Build history of the part. All positions in model axes, mm. A direction names the side the tool comes from. Give positions to 0.01 mm unless a question says otherwise; leave off trailing zeros. Order: outer loops, then holes, each group sorted by start corner. A loop starts at its lowest first (then second) coordinate and runs counter-clockwise, first axis right, second up. Notation, with made-up numbers: M 51.5,-24 L 92.5,-24 A10 cw 92.5,-6 Z; hole C 83.25,56.25 d2. An arc over 180 degrees is marked long. Use CSV: the item, a comma, the result in double quotes. Start each with the question number.
Item 1: Band-saw the part on A-A on x = 36. Write the cut outline in (y, z), plus the area to 3 significant figures.
Item 2: Band-saw the part on B-B on z = 47. Write the cut outline in (x, y), plus the area to 3 significant figures.
Item 3: Which spindle directions (+Z, -Z, +X, -X, +Y, -Y) get a long thin tool onto all of the face, cutting with end or side? Do faces 1 (the flat face through (103, -10, 10)), 2 (the cylindrical face through (25.945, -9.86, 38.974)), 3 (the flat face through (121, -13.31, 5)). Say none if no direction does.
Item 4: Wall check: line 1 along X through (y, z) = (-9.25, 3); line 2 along X through (y, z) = (-3.75, 21.5); line 3 along Z through (x, y) = (73, -15.25). Give the ranges that are in metal, low to high.
Item 5: Two-plate mould, pull along Y, no slides. Class faces 4 (the flat face through (3.41, -10.03, 2.91)), 5 (the flat face through (115, -5, 5)), 6 (the flat face through (52, -5.663, 28)), 7 (the flat face through (16.588, -9.86, 25.731)): pulls with the +Y half, pulls with the -Y half, needs draft (parallel to the pull), parting line crosses it, or undercut.
Item 6: Pin check, flat tips, straight feed: P1, Ø4, axis at x = 52, z = 29, coming from the +Y side; P2, Ø5, axis at x = 124.5, z = 4.5, coming from the +Y side; P3, Ø6, axis at x = 110.5, y = -12, coming from the +Z side; P4, Ø8, axis at y = -15.5, z = 42.5, coming from the -X side. Stop position of each tip, or through.
from build123d import *

# Parameters (mm, degrees)
F1_DEPTH  = 20
F4_DEPTH  = 50
F5_W      = 17
F5_H      = 6
F6_DEPTH  = 25
F8_R      = 4.25
F8_R_2    = 1.5
F9_DEPTH  = 25
F10_R     = 5.5
F11_DEPTH = 1.5


with BuildPart() as f1:
    # F0 (on Front) → F1 (new body)
    with BuildSketch(Plane.XZ):
        with BuildLine():
            Line((30, 51.9615242271), (0, 0))
            Line((0, 0), (130, 0))
            Line((130, 0), (130, 10))
            Line((130, 10), (85.1020127108, 10))
            ThreePointArc((85.1020127108, 10), (79.9256318088, 10.6814834742), (75.1020127108, 12.6794919243))
            Line((75.1020127108, 12.6794919243), (63.2290110083, 19.5343726533))
            ThreePointArc((63.2290110083, 19.5343726533), (61.9689506821, 21.9921089772), (62.2059384915, 24.7438459998))
            Line((62.2059384915, 24.7438459998), (44.644568833, 34.3145458549))
            ThreePointArc((44.644568833, 34.3145458549), (42.1322366307, 33.719194316), (39.6578564006, 34.4565538122))
            Line((39.6578564006, 34.4565538122), (26.1336276699, 42.2647709104))
            Line((26.1336276699, 42.2647709104), (31.2990381057, 51.2115242271))
            Line((31.2990381057, 51.2115242271), (30, 51.9615242271))
        make_face()
        with BuildLine():
            Line((10.4157161817, 11.1009099437), (10.4642531461, 15.1246181124))
            Line((10.4642531461, 15.1246181124), (22.8849254207, 36.637853556))
            ThreePointArc((22.8849254207, 36.637853556), (25.9989331967, 38.9877044803), (29.8532581245, 38.3851904586))
            Line((29.8532581245, 38.3851904586), (73.3850632782, 11.3456928945))
            ThreePointArc((73.3850632782, 11.3456928945), (77.1137537202, 5.8788979441), (72.1524804727, 1.5))
            Line((72.1524804727, 1.5), (24.9912310392, 1.5))
            Line((24.9912310392, 1.5), (10.4157161817, 11.1009099437))
        make_face(mode=Mode.SUBTRACT)
    extrude(amount=F1_DEPTH)

    # F3 (on face) → F4 (cut)
    with BuildSketch(Plane(origin=(70, 0, 70), x_dir=(0.7071067812, 0, -0.7071067812), z_dir=(0.7071067812, 0, 0.7071067812))):
        with BuildLine():
            ThreePointArc((13.0375107105, -5.6630554804), (9.0375107105, -9.6630554804), (13.0375107105, -13.6630554804))
            Line((13.0375107105, -13.6630554804), (21.0375107105, -13.6630554804))
            ThreePointArc((21.0375107105, -13.6630554804), (25.0375107105, -9.6630554804), (21.0375107105, -5.6630554804))
            Line((21.0375107105, -5.6630554804), (13.0375107105, -5.6630554804))
        make_face()
    extrude(amount=-F4_DEPTH, mode=Mode.SUBTRACT)

    # F5 (on Top) → F6 (cut)
    with BuildSketch(Plane.XY):
        with BuildLine():
            Line((130, 0), (95, 0))
            ThreePointArc((95, 0), (96.2962522412, -3.5190565155), (99.7416600585, -5))
            Line((99.7416600585, -5), (130, -5))
            Line((130, -5), (130, 0))
        make_face()
        with BuildLine():
            ThreePointArc((99.7416600585, -15), (96.2962522412, -16.4809434845), (95, -20))
            Line((95, -20), (130, -20))
            Line((130, -20), (130, -15))
            Line((130, -15), (99.7416600585, -15))
        make_face()
        with Locations((121.5, -10.3095373929)):
            Rectangle(F5_W, F5_H)
        with BuildLine():
            ThreePointArc((113, -7.3095373929), (110, -10.3095373929), (113, -13.3095373929))
            Line((113, -13.3095373929), (113, -7.3095373929))
        make_face()
    extrude(amount=F6_DEPTH, mode=Mode.SUBTRACT)

    # F8 (on face) → F9 (cut)
    with BuildSketch(Plane(origin=(0, 0, 0), x_dir=(0, 1, 0), z_dir=(0.8660254038, 0, -0.5))):
        with Locations((-10, 8.6775068194)):
            Circle(F8_R)
        with Locations((-5.6418100949, 25)):
            Circle(F8_R_2)
        with Locations((-15.6433817795, 25)):
            Circle(F8_R_2)
        with Locations((-5.5963639886, 31.9998524735)):
            Circle(F8_R_2)
        with Locations((-5.5509178823, 38.9997049471)):
            Circle(F8_R_2)
        with Locations((-15.5971498309, 31.9998473274)):
            Circle(F8_R_2)
        with Locations((-15.5509178823, 38.9996946548)):
            Circle(F8_R_2)
    extrude(amount=F9_DEPTH, mode=Mode.SUBTRACT)

    # F10 (on face) → F11 (cut)
    with BuildSketch(Plane(origin=(0, 0, 0), x_dir=(0, 1, 0), z_dir=(0.8660254038, 0, -0.5))):
        with Locations((-10, 8.6775068194)):
            Circle(F10_R)
    extrude(amount=F11_DEPTH, mode=Mode.SUBTRACT)


solid = f1.part
Model answer:
1,outline,"M -20,0 L 0,0 L 0,1.5 L -20,1.5 Z; M -20,34.57 L 0,34.57 L 0,36.57 L -20,36.57 Z"
1,area,"70.0 mm^2"
2,outline,"M 27.14,-20 L 28.87,-20 L 28.87,0 L 27.14,0 Z"
2,area,"34.6 mm^2"
3,face 1,"+Z, +X, +Y, -Y"
3,face 2,"+Y, -Y"
3,face 3,"+Z, -Z, +X"
4,line 1,"x = 3.46 to 3.79, 20.53 to 22.71, 75.72 to 110.19"
4,line 2,"x = 12.41 to 14.15, 57.04 to 62.09"
4,line 3,"z = 0 to 1.57, 11.58 to 13.89"
5,face 4,"undercut"
5,face 5,"pulls with the +Y half"
5,face 6,"undercut"
5,face 7,"needs draft"
6,P1,"stops at y = 0"
6,P2,"stops at y = -5"
6,P3,"stops at z = 10"
6,P4,"stops at x = 22.23"
